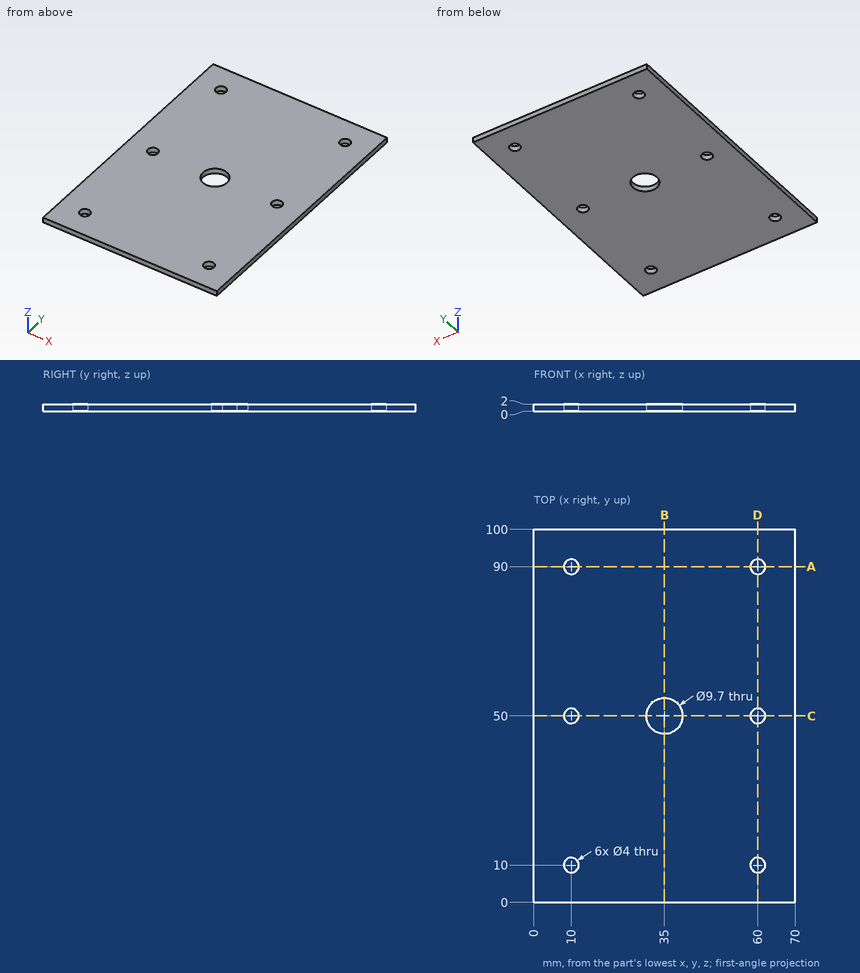
Source: three-view drawing plus pictorial views. Frame: mm from the lowest corner of the part. Give positions to 0.01 mm unless a question says otherwise; leave off trailing zeros. Order: outer loops, then holes, each group sorted by start corner. A loop starts at its lowest first (then second) coordinate and runs counter-clockwise, first axis right, second up. Notation, with made-up numbers: (20, -33) -> (53, -33) arc R25 cw to (53, -18) -> close; hole circle Ø5 at (50.5, 48). An arc over 180 degrees is marked (long way). Use a Markdown table: item, result.
Q1. Section B-B (x = 35). Return the cut outline in (y, z), and give its area (3 significant figures).
A:
| item | result |
|---|---|
| outline | (0, 0) -> (45.15, 0) -> (45.15, 2) -> (0, 2) -> close; (54.85, 0) -> (100, 0) -> (100, 2) -> (54.85, 2) -> close |
| area | 181 mm^2 |
Q2. Section C-C (y = 50). Return the cut outline in (x, z), and give its area (3 significant figures).
A:
| item | result |
|---|---|
| outline | (0, 0) -> (8, 0) -> (8, 2) -> (0, 2) -> close; (12, 0) -> (30.15, 0) -> (30.15, 2) -> (12, 2) -> close; (39.85, 0) -> (58, 0) -> (58, 2) -> (39.85, 2) -> close; (62, 0) -> (70, 0) -> (70, 2) -> (62, 2) -> close |
| area | 105 mm^2 |
Q3. Section A-A (y = 90). Return the cut outline in (x, z).
A:
| item | result |
|---|---|
| outline | (0, 0) -> (8, 0) -> (8, 2) -> (0, 2) -> close; (12, 0) -> (58, 0) -> (58, 2) -> (12, 2) -> close; (62, 0) -> (70, 0) -> (70, 2) -> (62, 2) -> close |
Q4. Material intervals for line 1 (Y direction, x = 10, z = 1.5); line 2 (X direction, y = 90, z = 0.95); line 3 (Y direction, x = 61.5, z = 1.85), sorted ascending. Write a range as [from, to].
A:
| item | result |
|---|---|
| line 1 | [0, 8], [12, 48], [52, 88], [92, 100] |
| line 2 | [0, 8], [12, 58], [62, 70] |
| line 3 | [0, 8.68], [11.32, 48.68], [51.32, 88.68], [91.32, 100] |
Q5. Section D-D (x = 60). Return the cut outline in (y, z), and give its area (3 significant figures).
A:
| item | result |
|---|---|
| outline | (0, 0) -> (8, 0) -> (8, 2) -> (0, 2) -> close; (12, 0) -> (48, 0) -> (48, 2) -> (12, 2) -> close; (52, 0) -> (88, 0) -> (88, 2) -> (52, 2) -> close; (92, 0) -> (100, 0) -> (100, 2) -> (92, 2) -> close |
| area | 176 mm^2 |
